```python
from build123d import *

# Parameters (mm, degrees)
F1_DEPTH = 50
F0_W     = 25
F0_H     = 20
F2_DEPTH = 25


with BuildPart() as f1:
    # F0 (on Front) → F1 (new body)
    with BuildSketch(Plane.XZ):
        Polygon((25, 0), (0, 0), (0, -22), (85, -22), (85, 0), (60, 0), align=None)
    extrude(amount=F1_DEPTH)

    # F0 (on Front) → F2 (join)
    with BuildSketch(Plane.XZ):
        with Locations((12.5, 10)):
            Rectangle(F0_W, F0_H)
        Polygon((25, 0), (0, 0), (0, -22), (85, -22), (85, 0), (60, 0), align=None)
        with Locations((72.5, 10)):
            Rectangle(F0_W, F0_H)
    extrude(amount=F2_DEPTH)


solid = f1.part
```
Geometry: final body of the model. Coordinates: model frame, mm. A direction names the side the tool comes from. Coordinates: 2 decimals unless noted, no trailing zeros. Order: outer loops, then holes, each group sorted by start corner. A loop starts at its lowest first (then second) coordinate and runs counter-clockwise, first axis right, second up. Notation, with made-up numbers: (28.25, -13.75) -> (66.25, -13.75) arc R17 ccw to (66.25, 17.25) -> close; hole circle Ø5 at (-4.75, 31.25). An arc over 180 degrees is marked (long way). Write item = value, one per line.
(1) Cut plane A-A on z = 5.5. Return loops of the section in (x, y).
Solved:
outline = (0, -25) -> (25, -25) -> (25, 0) -> (0, 0) -> close; (60, -25) -> (85, -25) -> (85, 0) -> (60, 0) -> close
(2) Cut plane C-C on x = 30. Return loops of the section in (y, z), plus the area to 3 significant figures.
Solved:
outline = (-50, -22) -> (0, -22) -> (0, 0) -> (-50, 0) -> close
area = 1,100 mm²
(3) Pull-direction query (X, two-part tool) for faces 1 (the flat face through (85, -19, -6)), 2 (the flat face through (60, -12, 10)), 3 (the flat face through (12, -12, 20)); classes: pulls with the +X half, pulls with the -X half, needs draft (parallel to the pull), parting line crosses it, or undercut.
Solved:
face_1 = pulls with the +X half
face_2 = undercut
face_3 = needs draft
(4) Cut plane D-D on x = 20.5. Return loops of the section in (y, z).
Solved:
outline = (-50, -22) -> (0, -22) -> (0, 20) -> (-25, 20) -> (-25, 0) -> (-50, 0) -> close
(5) Cut plane B-B on y = -10. Return loops of the section in (x, z), plus the area to 3 significant figures.
Solved:
outline = (0, -22) -> (85, -22) -> (85, 20) -> (60, 20) -> (60, 0) -> (25, 0) -> (25, 20) -> (0, 20) -> close
area = 2,870 mm²
(6) Access query for faces 4 (the flat face through (25, -12, 10)), 5 (the flat face through (72, -12, 20)), 6 (the flat face through (72, -25, 10)). Directions: +Z, -Z, +X, -X, +Y, -Y. A direction counts if a zero-diameter tool reaches every point of the face in a straight line with its end or side. Return the directions, or none.
Solved:
face_4 = +Z, +Y, -Y
face_5 = +Z, +X, -X, +Y, -Y
face_6 = +Z, +X, -X, -Y
(7) Line query: line 1 (X direction, y = -3.5, z = 3); line 2 (Z direction, x = 28.5, y = -8.5); line 3 (Y direction, x = 72, z = 11). Output: solid intervals per line, ascending.
Solved:
line_1 = 0 to 25, 60 to 85
line_2 = -22 to 0
line_3 = -25 to 0
(8) Pin query (flat end, axial travel): pin 1 Ø1 at (x, y) = (39.5, -27) entering from +Z; pin 2 Ø6 at (x, z) = (70.5, 13.5) entering from -Y. Return the tip coordinate at first contact, or that it passes through.
Solved:
pin_1 = 0
pin_2 = -25
